Geometry check sheet. Reference: the model listing, model coordinates, mm. Face numbers are marked on the shaded views. A direction names the side the tool comes from. Give positions to 0.01 mm unless a question says otherwise; leave off trailing zeros. Write each loop counter-clockwise with the first axis right and the second up, starting at its lowest first coordinate (ties: lowest second). Pieces come first, ordered by that corner, then holes. Notation, with made-up numbers: (-36, 0) - (-23, 0) arc R29 cw to (-23, 21) - close; hole circle Ø8 at (5.25, -10.75). An arc over 180 degrees is marked (long way). Write item = value, one per line. Start each with the question number.
(1) Section check C-C, the plane x = 26.5. Enter the section's corners in (y, z), plus the area to 3 significant figures.
(2) Section check B-B, the plane z = 30. Enter the section's corners in (x, y).
(3) Access from +Z, -Z, +X, -X, +Y, -Y to the whole of each face (thin tool, end or side, straight path). Record for the marked faces 1 and 2.
(4) Thickness scan on L1, parallel to X at y = -5, z = -27; L2, parallel to Z at x = 40, y = -4; L3, parallel to Y at x = 7.5, z = 25.5. Record the ranges inside material, lowest first.
(5) Draft check along Z on the marked faces 3, 4 and 5. Enter one of: pulls with the +Z half, pulls with the -Z half, needs draft (parallel to the pull), parting line crosses it, or undercut.
(6) Section check A-A, the plane x = 37.5. Enter the section's corners in (y, z).
(7) Section check D-D, the plane z = -29. Give the number of separate pieces and of enclosed holes in the cut face, plus the area to 3 significant figures.
(8) Depth check by flat-ended pin: pin 1 Ø5 at (x, y) = (14, -6) entering from -Z; pin 2 Ø5 at (y, z) = (31.5, 5.5) entering from -X; pin 3 Ø11.5 at (x, z) = (-40, -27.5) entering from +Y. Enter the tip coordinate at first touch or a pass-through.
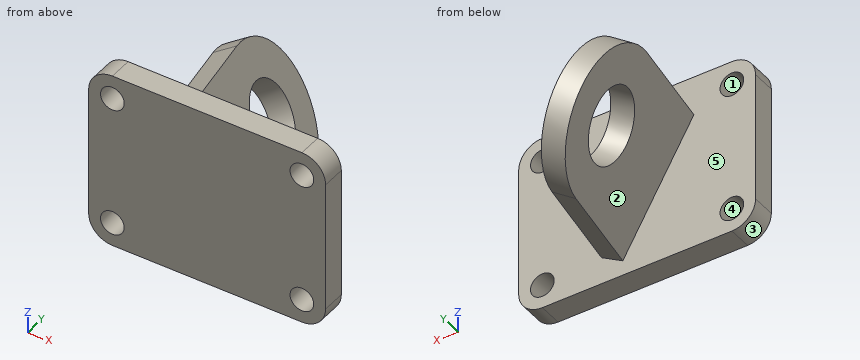
```python
from build123d import *

# Parameters (mm, degrees)
SKETCH_1_R      = 5
EXTRUDE_1_DEPTH = 10
SKETCH_3_R      = 15
EXTRUDE_2_DEPTH = 10


with BuildPart() as part:
    # Sketch 1 → Extrude 1 (new body)
    with BuildSketch(Plane(origin=(0, 0, 0), x_dir=(1, 0, 0), z_dir=(0, 1, 0))):
        with BuildLine():
            Line((-40, -37.5), (40, -37.5))
            ThreePointArc((40, -37.5), (47.071067812, -34.571067812), (50, -27.5))
            Line((50, -27.5), (50, 27.5))
            ThreePointArc((50, 27.5), (47.071067812, 34.571067812), (40, 37.5))
            Line((40, 37.5), (-40, 37.5))
            ThreePointArc((-40, 37.5), (-47.071067812, 34.571067812), (-50, 27.5))
            Line((-50, 27.5), (-50, -27.5))
            ThreePointArc((-50, -27.5), (-47.071067812, -34.571067812), (-40, -37.5))
        make_face()
        with Locations((-40, 27.5)):
            Circle(SKETCH_1_R, mode=Mode.SUBTRACT)
        with Locations((40, 27.5)):
            Circle(SKETCH_1_R, mode=Mode.SUBTRACT)
        with Locations((-40, -27.5)):
            Circle(SKETCH_1_R, mode=Mode.SUBTRACT)
        with Locations((40, -27.5)):
            Circle(SKETCH_1_R, mode=Mode.SUBTRACT)
    extrude(amount=-EXTRUDE_1_DEPTH)

    # Sketch 3 → Extrude 2 (add)
    with BuildSketch(Plane(origin=(0, 0, 0), x_dir=(0.5, 0, -0.866025404), z_dir=(0.836516304, 0.258819045, 0.482962913))):
        with BuildLine():
            Line((-30, 50), (-30, 0))
            Line((-30, 0), (30, 0))
            Line((30, 0), (30, 50))
            ThreePointArc((30, 50), (0, 80), (-30, 50))
        make_face()
        with Locations((0, 50)):
            Circle(SKETCH_3_R, mode=Mode.SUBTRACT)
    extrude(amount=-EXTRUDE_2_DEPTH)


solid = part.part
```
Model answer:
q1.outline = (-10, -37.5) - (0, -37.5) - (0, 37.5) - (-10, 37.5) - close
q1.area = 750 mm²
q2.outline = (-49.68, -10) - (-44.33, -10) - (-44.33, 0) - (-49.68, 0) - close; (-35.67, -10) - (35.67, -10) - (35.67, 0) - (-35.67, 0) - close; (44.33, -10) - (49.68, -10) - (49.68, 0) - (44.33, 0) - close
q3.face_1 = +Y, -Y
q3.face_2 = -Z, -X
q4.L1 = -50 to -44.97, -35.03 to 35.03, 44.97 to 50
q4.L2 = -37.5 to -32.5, -22.5 to 22.5, 32.5 to 37.5
q4.L3 = -10 to 0
q5.face_3 = pulls with the -Z half
q5.face_4 = undercut
q5.face_5 = needs draft
q6.outline = (-10, -37.5) - (0, -37.5) - (0, -31.83) - (-10, -31.83) - close; (-10, -23.17) - (0, -23.17) - (0, 23.17) - (-10, 23.17) - close; (-10, 31.83) - (0, 31.83) - (0, 37.5) - (-10, 37.5) - close
q7.separate_pieces = 3
q7.enclosed_holes = 0
q7.area = 1,550 mm²
q8.pin_1 = -37.5
q8.pin_2 = -26.51
q8.pin_3 = 0
